Job drawing, mm, ordinate dimensions from the low corner. One solid piece. A direction names the side the tool comes from. Coordinates: 2 decimals unless noted, no trailing zeros. Loops run counter-clockwise (first coordinate to the right, second up) from the corner with the lowest first, then second, coordinate; pieces in that order, holes last. Notation, with made-up numbers: (56, -29.75) - (97, -29.75) arc R14 ccw to (97, -8.75) - close; hole circle Ø11 at (53.5, 39.25). An arc over 180 degrees is marked (long way). Use a Markdown table: item, result. Add a question column.
1. Band-saw the part on D-D, the plane x = 26. Give the cut face in (y, z), plus the area to 3 significant figures.
2. 3-axis set-ups, long thin cutter, end or side, ignore diameter. For the marked faces 1 and 2: which of +Z, -Z, +X, -X, +Y, -Y reach the whole face in a straight line?
3. Band-saw the part on B-B, the plane z = 7.5. Give the cut face in (x, y).
4. Wall check: probe 1 along X at (y, z) = (0.5, 7.5); probe 2 along Z at (x, y) = (14.5, 0.45); probe 3 along Y at (x, z) = (6.5, 16.05). Give the ranges that are in metal, low to high. Write a range as [from, to].
5. Band-saw the part on C-C, the plane x = 45.5. Give the cut face in (y, z).
6. Band-saw the part on A-A, the plane x = 89.5. Give the cut face in (y, z).
7. Drop flat-ended pins along their axis: pin 1 (6 mm diameter, centred on y = 11.5, z = 10.5, fed in from +X); pin 2 (6 mm diameter, centred on x = 14.5, z = 7.5, fed in from +Y) (1 decimal); pin 3 (2 mm diameter, centred on x = 84.5, y = 9.5, fed in from -Z); pin 4 (4.5 mm diameter, centred on x = 28.5, z = 9.5, fed in from +Y). Give the stop position or say it passes through.
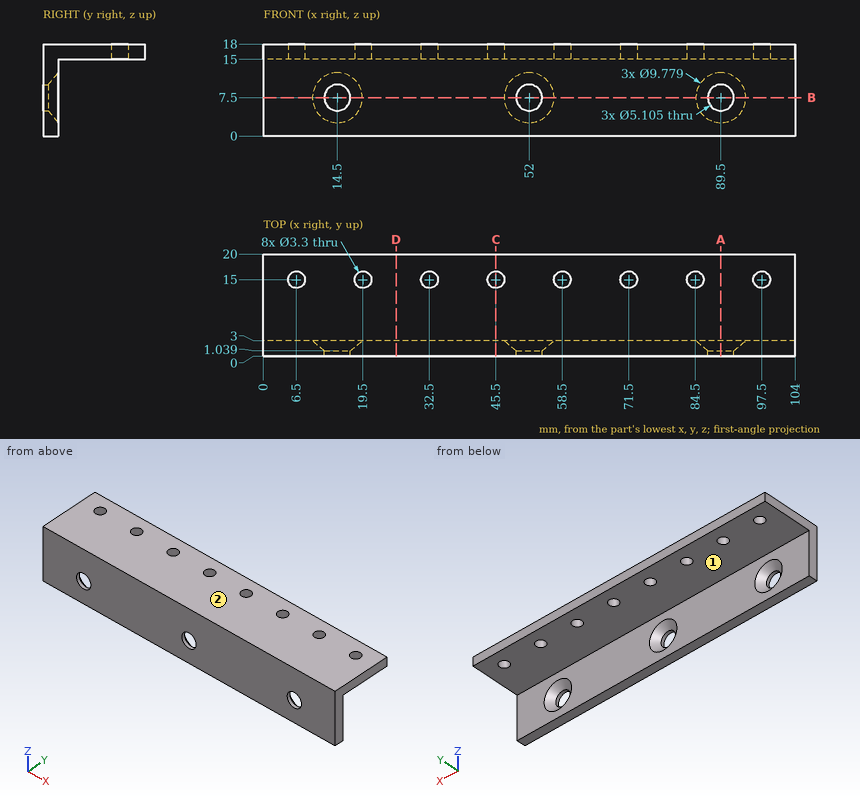
Geometry check:
| question | item | result |
|---|---|---|
| 1 | outline | (0, 0) - (3, 0) - (3, 15) - (20, 15) - (20, 18) - (0, 18) - close |
| 1 | area | 105 mm^2 |
| 2 | face 1 | -Z, +X, -X, +Y |
| 2 | face 2 | +Z, +X, -X, +Y, -Y |
| 3 | outline | (0, 0) - (11.95, 0) - (11.95, 1.04) - (9.61, 3) - (0, 3) - close; (17.05, 0) - (49.45, 0) - (49.45, 1.04) - (47.11, 3) - (19.39, 3) - (17.05, 1.04) - close; (54.55, 0) - (86.95, 0) - (86.95, 1.04) - (84.61, 3) - (56.89, 3) - (54.55, 1.04) - close; (92.05, 0) - (104, 0) - (104, 3) - (94.39, 3) - (92.05, 1.04) - close |
| 4 | probe 1 | x = [0, 11.95], [17.05, 49.45], [54.55, 86.95], [92.05, 104] |
| 4 | probe 2 | z = [0, 4.95], [10.05, 18] |
| 4 | probe 3 | y = [0, 13.35], [16.65, 20] |
| 5 | outline | (0, 0) - (3, 0) - (3, 15) - (13.35, 15) - (13.35, 18) - (0, 18) - close; (16.65, 15) - (20, 15) - (20, 18) - (16.65, 18) - close |
| 6 | outline | (0, 0) - (3, 0) - (3, 2.61) - (1.04, 4.95) - (0, 4.95) - close; (0, 10.05) - (1.04, 10.05) - (3, 12.39) - (3, 15) - (20, 15) - (20, 18) - (0, 18) - close |
| 7 | pin 1 | passes through |
| 7 | pin 2 | stops at y = 1.4 |
| 7 | pin 3 | stops at z = 15 |
| 7 | pin 4 | stops at y = 3 |
